Read the model definition and answer for the solid it produces. Units are mm, in the model's axes. Give positions to 0.01 mm unless a question says otherwise; leave off trailing zeros. Order: outer loops, then holes, each group sorted by start corner. A loop starts at its lowest first (then second) coordinate and runs counter-clockwise, first axis right, second up. Notation, with made-up numbers: (39.25, 10) - (67.25, 10) arc R29 cw to (67.25, 33) - close; hole circle Ø3 at (13.5, -11.75). An arc over 180 degrees is marked (long way). Use a Markdown table: item, result. Add a question column.
1. Consider L1, parallel to X at y = 25.5, z = 1.2; L2, parallel to X at y = 17.5, z = 1.1; L3, parallel to X at y = 11, z = 1.2. Determine where each line is inside the solid, lowest interval first.
2. A cutting plane is placed at A-A on x = 24.5. Determine the outline of the cut face in (y, z).
3. A cutting plane is placed at B-B on y = 26. Determine the outline of the cut face in (x, z), and give its area (3 significant figures).
4. A flat-ended cylindrical pin translates along its axis: P1, Ø1.2, axis at x = 21.8, y = 21.89, coming from the -Z side. Find the tip coordinate at first contact, or state that the pin passes through.
5. A cutting plane is placed at C-C on z = 0.6. State how many separate pieces and enclosed holes the cut face has, and give its area (3 significant figures).
```python
from build123d import *

# Parameters (mm, degrees)
F0_W     = 6
F0_H     = 6
F0_W_2   = 4
F0_H_2   = 4
F0_W_3   = 2
F0_H_3   = 2
F0_R     = 1
F0_R_2   = 2
F0_R_3   = 3
F1_DEPTH = 2


with BuildPart() as f1:
    # F0 (on Top) → F1 (new body)
    with BuildSketch(Plane.XY):
        with BuildLine():
            ThreePointArc((0, 5), (1.464466, 1.464466), (5, 0))
            Line((5, 0), (40, 0))
            Line((40, 0), (40, 30))
            Line((40, 30), (0, 30))
            Line((0, 30), (0, 5))
        make_face()
        with BuildLine():
            Line((5, 4.231699), (5, 4.331699))
            Line((5, 4.331699), (34.911151, 4.331699))
            ThreePointArc((34.911151, 4.331699), (34.946507, 4.317055), (34.961151, 4.281699))
            ThreePointArc((34.961151, 4.281699), (34.946507, 4.246344), (34.911151, 4.231699))
            Line((34.911151, 4.231699), (5, 4.231699))
        make_face(mode=Mode.SUBTRACT)
        with BuildLine():
            Line((5, 8.531699), (5, 8.831699))
            Line((5, 8.831699), (34.834979, 8.831699))
            ThreePointArc((34.834979, 8.831699), (34.941045, 8.787765), (34.984979, 8.681699))
            ThreePointArc((34.984979, 8.681699), (34.941045, 8.575633), (34.834979, 8.531699))
            Line((34.834979, 8.531699), (5, 8.531699))
        make_face(mode=Mode.SUBTRACT)
        with BuildLine():
            Line((5, 13.331699), (5, 14.331699))
            Line((5, 14.331699), (34.378945, 14.331699))
            ThreePointArc((34.378945, 14.331699), (34.732499, 14.185253), (34.878945, 13.831699))
            ThreePointArc((34.878945, 13.831699), (34.732499, 13.478146), (34.378945, 13.331699))
            Line((34.378945, 13.331699), (5, 13.331699))
        make_face(mode=Mode.SUBTRACT)
        with BuildLine():
            Line((5, 6.331699), (5, 6.531699))
            Line((5, 6.531699), (34.911151, 6.531699))
            ThreePointArc((34.911151, 6.531699), (34.981862, 6.50241), (35.011151, 6.431699))
            ThreePointArc((35.011151, 6.431699), (34.981862, 6.360989), (34.911151, 6.331699))
            Line((34.911151, 6.331699), (5, 6.331699))
        make_face(mode=Mode.SUBTRACT)
        with BuildLine():
            Line((5, 10.831699), (5, 11.331699))
            Line((5, 11.331699), (34.814051, 11.331699))
            ThreePointArc((34.814051, 11.331699), (34.990828, 11.258476), (35.064051, 11.081699))
            ThreePointArc((35.064051, 11.081699), (34.990828, 10.904923), (34.814051, 10.831699))
            Line((34.814051, 10.831699), (5, 10.831699))
        make_face(mode=Mode.SUBTRACT)
        with Locations((6.205281, 24.370336)):
            Rectangle(F0_W, F0_H, mode=Mode.SUBTRACT)
        with Locations((14.165812, 25.370336)):
            Rectangle(F0_W_2, F0_H_2, mode=Mode.SUBTRACT)
        with Locations((19.510129, 26.370336)):
            Rectangle(F0_W_3, F0_H_3, mode=Mode.SUBTRACT)
        with BuildLine():
            Line((5, 16.331699), (5, 17.831699))
            Line((5, 17.831699), (34.25, 17.831699))
            ThreePointArc((34.25, 17.831699), (34.78033, 17.612029), (35, 17.081699))
            ThreePointArc((35, 17.081699), (34.78033, 16.551369), (34.25, 16.331699))
            Line((34.25, 16.331699), (5, 16.331699))
        make_face(mode=Mode.SUBTRACT)
        with Locations((21.798409, 21.888405)):
            Circle(F0_R, mode=Mode.SUBTRACT)
        with Locations((27.244295, 23.247146)):
            Circle(F0_R_2, mode=Mode.SUBTRACT)
        with Locations((34.282601, 24.221355)):
            Circle(F0_R_3, mode=Mode.SUBTRACT)
    extrude(amount=F1_DEPTH)


solid = f1.part
```
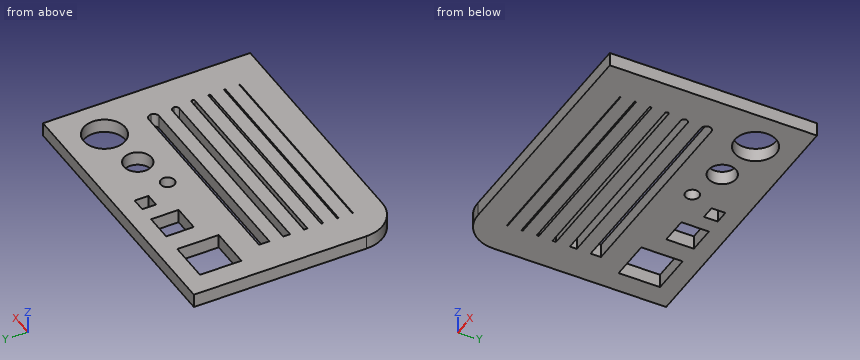
Output values:
| question | item | result |
|---|---|---|
| 1 | L1 | 0 to 3.21, 9.21 to 12.17, 16.17 to 18.51, 20.51 to 31.57, 37 to 40 |
| 1 | L2 | 0 to 5, 34.87 to 40 |
| 1 | L3 | 0 to 5, 35.05 to 40 |
| 2 | outline | (0, 0) - (4.23, 0) - (4.23, 2) - (0, 2) - close; (4.33, 0) - (6.33, 0) - (6.33, 2) - (4.33, 2) - close; (6.53, 0) - (8.53, 0) - (8.53, 2) - (6.53, 2) - close; (8.83, 0) - (10.83, 0) - (10.83, 2) - (8.83, 2) - close; (11.33, 0) - (13.33, 0) - (13.33, 2) - (11.33, 2) - close; (14.33, 0) - (16.33, 0) - (16.33, 2) - (14.33, 2) - close; (17.83, 0) - (30, 0) - (30, 2) - (17.83, 2) - close |
| 3 | outline | (0, 0) - (3.21, 0) - (3.21, 2) - (0, 2) - close; (9.21, 0) - (12.17, 0) - (12.17, 2) - (9.21, 2) - close; (16.17, 0) - (18.51, 0) - (18.51, 2) - (16.17, 2) - close; (20.51, 0) - (31.87, 0) - (31.87, 2) - (20.51, 2) - close; (36.7, 0) - (40, 0) - (40, 2) - (36.7, 2) - close |
| 3 | area | 46.3 mm² |
| 4 | P1 | through |
| 5 | separate pieces | 1 |
| 5 | enclosed holes | 12 |
| 5 | area | 987 mm² |
